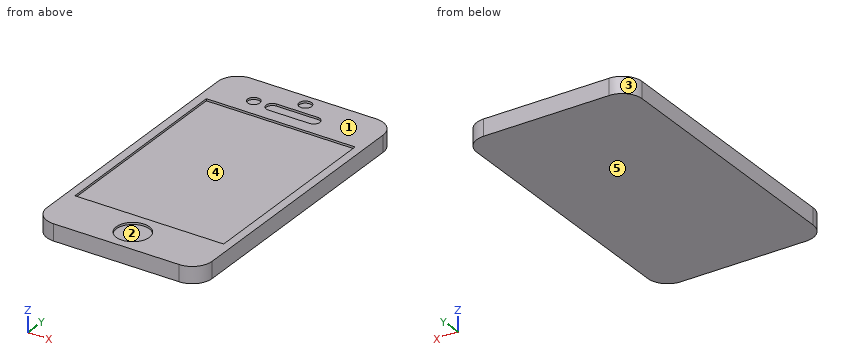
```python
from build123d import *

# Parameters (mm, degrees)
F3_DEPTH = 6.35
F0_R     = 6.35
F0_W     = 57.15
F0_H     = 76.2
F0_R_2   = 2.38125
F1_DEPTH = 0.79375


with BuildPart() as f3:
    # F2 (on Top) → F3 (new body)
    with BuildSketch(Plane.XY):
        with BuildLine():
            ThreePointArc((31.75, 49.53), (29.518154, 54.918154), (24.13, 57.15))
            Line((24.13, 57.15), (-24.13, 57.15))
            ThreePointArc((-24.13, 57.15), (-29.518154, 54.918154), (-31.75, 49.53))
            Line((-31.75, 49.53), (-31.75, -49.53))
            ThreePointArc((-31.75, -49.53), (-29.518154, -54.918154), (-24.13, -57.15))
            Line((-24.13, -57.15), (24.13, -57.15))
            ThreePointArc((24.13, -57.15), (29.518154, -54.918154), (31.75, -49.53))
            Line((31.75, -49.53), (31.75, 49.53))
        make_face()
    extrude(amount=F3_DEPTH)

    # F0 (on face) → F1 (cut)
    with BuildSketch(Plane.XY.offset(6.35)):
        with Locations((0, -47.625)):
            Circle(F0_R)
        with BuildLine():
            ThreePointArc((-7.9375, 47.625), (-10.31875, 45.24375), (-7.9375, 42.8625))
            Line((-7.9375, 42.8625), (7.9375, 42.8625))
            ThreePointArc((7.9375, 42.8625), (10.31875, 45.24375), (7.9375, 47.625))
            Line((7.9375, 47.625), (-7.9375, 47.625))
        make_face()
        Rectangle(F0_W, F0_H)
        with Locations((-15.093792, 45.24375)):
            Circle(F0_R_2)
        with Locations((0, 52.3875)):
            Circle(F0_R_2)
    extrude(amount=-F1_DEPTH, mode=Mode.SUBTRACT)


solid = f3.part
```
For this review, take the finished solid that the model builds, in its own axes (mm). Face numbers are marked on the shaded views. A direction names the side the tool comes from. Round coordinates to 2 decimals unless told otherwise and drop trailing zeros. Write each loop counter-clockwise with the first axis right and the second up, starting at its lowest first coordinate (ties: lowest second). Pieces come first, ordered by that corner, then holes. Notation, with made-up numbers: (-15.5, -2) - (32.5, -2) arc R12 ccw to (32.5, 4) - close; hole circle Ø8 at (18.5, 30). An arc over 180 degrees is marked (long way). Answer as CSV lines item,"result". Start each with the question number.
(1) For line 1 (X direction, y = -50, z = 3); line 2 (Z direction, x = -19.5, y = 6.5); line 3 (X direction, y = -52, z = 2.5), list the stretches that pass through material, from the lowest coordinate up.
(2) Add section B-B, the plane y = -7.5. State the section outline as (x, z) points (3 decimals), plus the area to 3 significant figures.
(3) Mouldability with a two-part tool opening along X and no side actions: class the marked faces 3, 4 and 5 as +X half, -X half, draft (parallel to the pull), parting line (faces both ways), or undercut.
(4) For pin 1 (4 mm diameter, centred on x = 25, y = 4, fed in from +Z), flat-tipped, find the tip position at first contact; note if it passes through.
(5) Machinability: for the marked faces 1 and 2, which of the approach directions +Z, -Z, +X, -X, +Y, -Y give a long, thin tool a straight path to every point of the face, cutting with its end or side? Answer none if there is none.
(6) Add section A-A, the plane x = 16. State the section outline as (y, z) points.
From the geometry:
1,line 1,"x = -31.74 to 31.74"
1,line 2,"z = 0 to 5.56"
1,line 3,"x = -31.34 to 31.34"
2,outline,"(-31.75, 0) - (31.75, 0) - (31.75, 6.35) - (28.575, 6.35) - (28.575, 5.556) - (-28.575, 5.556) - (-28.575, 6.35) - (-31.75, 6.35) - close"
2,area,"358 mm²"
3,face 3,"-X half"
3,face 4,"undercut"
3,face 5,"draft"
4,pin 1,"stops at z = 5.56"
5,face 1,"+Z, +X, -X, +Y, -Y"
5,face 2,"+Z"
6,outline,"(-57.15, 0) - (57.15, 0) - (57.15, 6.35) - (38.1, 6.35) - (38.1, 5.56) - (-38.1, 5.56) - (-38.1, 6.35) - (-57.15, 6.35) - close"
